Check sheet for the drawn part. Datum: minimum x, y, z corner. Units: mm. Give positions to 0.01 mm unless a question says otherwise; leave off trailing zeros. Write each loop counter-clockwise with the first axis right and the second up, starting at its lowest first coordinate (ties: lowest second). Pieces come first, ordered by that corner, then holes. Notation, with made-up numbers: (47.25, 60) - (80.25, 60) arc R27 ccw to (80.25, 76) - close; hole circle Ø9 at (20, -28.75). An arc over 180 degrees is marked (long way). Answer as a JSON object with one key per item and string values. Group by question number.
Item 1: Scan lines: line 1 along Z through (x, y) = (10, 58); line 2 along X through (y, z) = (36, 5.5); line 3 along X through (y, z) = (113, 12.75). Record each from-to range of solid material in increasing order. Write a range as [from, to].
Item 2: Sectioned sample at B-B, the plane z = 12.25. Record the boundary of the cut face in (x, y), and give its area (3 significant figures).
Item 3: Sectioned sample at A-A, the plane x = 7. Record the boundary of the cut face in (y, z), and give its area (3 significant figures).
Item 4: Sectioned sample at D-D, the plane x = 30. Record the boundary of the cut face in (y, z), and give its area (3 significant figures).
Item 5: Go/stop test with a flat-tipped pin: pin 1 (6 mm diameter, centred on x = 10, z = 10, fed in from -Y). Record where the tip stops, or that it passes through.
Item 6: Sectioned sample at C-C, the plane y = 27. Record the boundary of the cut face in (x, z).
Item 7: Draft check along Z on the marked faces 1, 2 and 3. Enter one of: +Z half, -Z half, draft (parallel to the pull), parting line (faces both ways), or undercut.
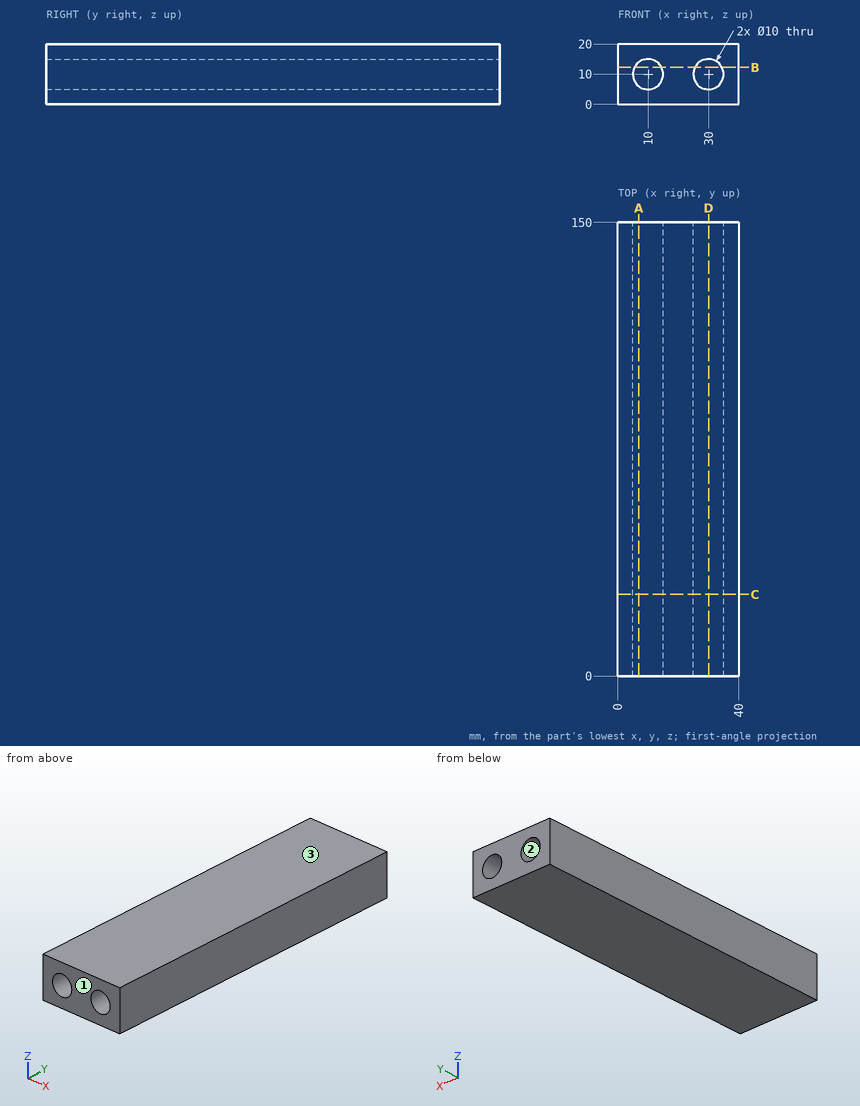
Geometry check:
{
 "1": {"line 1": "[0, 5], [15, 20]", "line 2": "[0, 7.82], [12.18, 27.82], [32.18, 40]", "line 3": "[0, 5.82], [14.18, 25.82], [34.18, 40]"},
 "2": {"outline": "(0, 0) - (5.53, 0) - (5.53, 150) - (0, 150) - close; (14.47, 0) - (25.53, 0) - (25.53, 150) - (14.47, 150) - close; (34.47, 0) - (40, 0) - (40, 150) - (34.47, 150) - close", "area": "3,320 mm^2"},
 "3": {"outline": "(0, 0) - (150, 0) - (150, 6) - (0, 6) - close; (0, 14) - (150, 14) - (150, 20) - (0, 20) - close", "area": "1,800 mm^2"},
 "4": {"outline": "(0, 0) - (150, 0) - (150, 5) - (0, 5) - close; (0, 15) - (150, 15) - (150, 20) - (0, 20) - close", "area": "1,500 mm^2"},
 "5": {"pin 1": "through"},
 "6": {"outline": "(0, 0) - (40, 0) - (40, 20) - (0, 20) - close; hole circle Ø10 at (10, 10); hole circle Ø10 at (30, 10)"},
 "7": {"face 1": "draft", "face 2": "undercut", "face 3": "+Z half"}
}
